```python
from build123d import *

# Parameters (mm, degrees)
SKETCH1_R            = 6.5
BOSS_EXTRUDE1_DEPTH  = 4
SKETCH4_R            = 2.6
CUT_EXTRUDE1_DEPTH   = 10
SKETCH5_W            = 200
SKETCH5_H            = 4
BOSS_EXTRUDE2_DEPTH  = 100
SKETCH8_R            = 2.6
CUT_EXTRUDE2_DEPTH   = 100
SKETCH9_R            = 5
SKETCH9_R_2          = 1.75
CUT_EXTRUDE3_DEPTH   = 10
CONVERT_SOLID3_START = -100
CONVERT_SOLID3_DEPTH = 200
SKETCH11_R           = 2.6
CUT_EXTRUDE4_DEPTH   = 10


# Read off the part's stored shape, not the designer's step: Convert-Solid3
with BuildPart() as part:
    # Sketch1 → Boss-Extrude1 (new body)
    with BuildSketch(Plane.XY):
        with BuildLine():
            Line((100, -4), (100, 0))
            Line((100, 0), (36.695562583, 145.919663525))
            ThreePointArc((36.695562583, 145.919663525), (0, 170), (-36.695562583, 145.919663525))
            Line((-36.695562583, 145.919663525), (-100, 0))
            Line((-100, 0), (-100, -4))
            Line((-100, -4), (100, -4))
        make_face()
        with Locations((0, 130)):
            Circle(SKETCH1_R, mode=Mode.SUBTRACT)
    extrude(amount=BOSS_EXTRUDE1_DEPTH)

    # Sketch4 → Cut-Extrude1 (cut)
    with BuildSketch(Plane(origin=(0, 0, 0), x_dir=(-1, 0, 0), z_dir=(0, 0, -1))):
        with Locations((0, 111.75)):
            Circle(SKETCH4_R)
        with Locations((0, 148.25)):
            Circle(SKETCH4_R)
    extrude(amount=-CUT_EXTRUDE1_DEPTH, mode=Mode.SUBTRACT)

    # Sketch5 → Boss-Extrude2 (add)
    with BuildSketch(Plane(origin=(0, 0, 0), x_dir=(-1, 0, 0), z_dir=(0, 0, -1))):
        with Locations((0, -2)):
            Rectangle(SKETCH5_W, SKETCH5_H)
    extrude(amount=-BOSS_EXTRUDE2_DEPTH)

    # Sketch8 → Cut-Extrude2 (cut)
    with BuildSketch(Plane(origin=(0, 0, 0), x_dir=(1, 0, 0), z_dir=(0, 1, 0))):
        with Locations(Location((-85, -80, 0), (0, 0, 270))):
            Circle(SKETCH8_R)
        with Locations(Location((-85, -20, 0), (0, 0, 270))):
            Circle(SKETCH8_R)
        with Locations(Location((85, -80, 0), (0, 0, 270))):
            Circle(SKETCH8_R)
        with Locations(Location((85, -20, 0), (0, 0, 270))):
            Circle(SKETCH8_R)
    extrude(amount=-CUT_EXTRUDE2_DEPTH, mode=Mode.SUBTRACT)

    # Sketch9 → Cut-Extrude3 (cut)
    with BuildSketch(Plane.XY.offset(4)):
        with Locations((0, 25)):
            Circle(SKETCH9_R)
        with Locations((0, 33)):
            Circle(SKETCH9_R_2)
        with Locations((0, 17)):
            Circle(SKETCH9_R_2)
        with Locations((8, 25)):
            Circle(SKETCH9_R_2)
        with Locations((-8, 25)):
            Circle(SKETCH9_R_2)
    extrude(amount=-CUT_EXTRUDE3_DEPTH, mode=Mode.SUBTRACT)

    # Convert-Solid3 outline → Convert-Solid3 (cut)
    with BuildSketch(Plane.YZ.offset(CONVERT_SOLID3_START)):
        with BuildLine():
            ThreePointArc((-0.2, 0), (-2.887005769, 1.112994231), (-4, 3.8))
            Line((-4, 3.8), (-3.999999957, 100))
            Line((-3.999999957, 100), (-6, 100))
            Line((-6, 100), (-6, -1))
            Line((-6, -1), (171, -1))
            Line((171, -1), (171, 7.6e-08))
            Line((171, 7.6e-08), (-0.2, 0))
        make_face()
        with BuildLine():
            Line((0, 100), (-2, 100))
            Line((-2, 100), (-2, 3.8))
            ThreePointArc((-2, 3.8), (-1.472792206, 2.527207794), (-0.2, 2))
            Line((-0.2, 2), (171, 2))
            Line((171, 2), (171, 4))
            Line((171, 4), (0, 4))
            Line((0, 4), (0, 100))
        make_face()
    extrude(amount=CONVERT_SOLID3_DEPTH, mode=Mode.SUBTRACT)

    # Sketch11 → Cut-Extrude4 (cut)
    with BuildSketch(Plane.XY.offset(2)):
        with Locations((0, 70)):
            Circle(SKETCH11_R)
        with Locations((0, 96.75)):
            Circle(SKETCH11_R)
        with Locations((-15, 96.75)):
            Circle(SKETCH11_R)
        with Locations((-15, 70)):
            Circle(SKETCH11_R)
    extrude(amount=-CUT_EXTRUDE4_DEPTH, mode=Mode.SUBTRACT)


solid = part.part
```
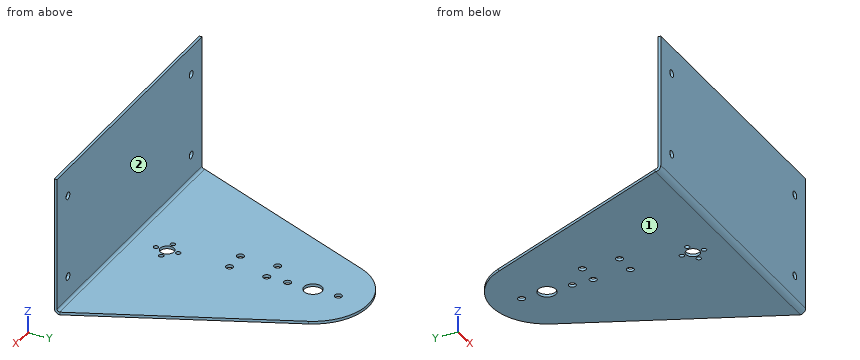
Geometry: final body of the model. Coordinates: model frame, mm. Face numbers are marked on the shaded views. A direction names the side the tool comes from. Coordinates: 2 decimals unless noted, no trailing zeros. Order: outer loops, then holes, each group sorted by start corner. A loop starts at its lowest first (then second) coordinate and runs counter-clockwise, first axis right, second up.
Item 1: Material intervals for line 1 along X through (y, z) = (-3.35, 20); line 2 along Y through (x, z) = (-15, 0.5); line 3 along Y through (x, z) = (-15, 1), sorted ascending.
Answer:
line 1: x = -100 to -87.6, -82.4 to 82.4, 87.6 to 100
line 2: y = -2.08 to 67.4, 72.6 to 94.15, 99.35 to 167.08
line 3: y = -2.77 to 67.4, 72.6 to 94.15, 99.35 to 167.08
Item 2: Contact query for flat-ended pins moving along their axis: P1, Ø6, axis at x = -15, y = 96.75, coming from the +Z side; P2, Ø10, axis at x = 22, z = 30.5, coming from the +Y side. Output: stop coordinate, or through.
Answer:
P1: stops at z = 2
P2: stops at y = -2
Item 3: Section query D-D (x = 85). Output: boundary loops of the cut face in (y, z), then the cut area to 3 significant figures.
Answer:
outline: (-4, 3.8) arc R3.8 ccw to (-0.2, 0) - (34.58, 0) - (34.58, 2) - (-0.2, 2) arc R1.8 cw to (-2, 3.8) - (-2, 17.4) - (-4, 17.4) - close; (-4, 22.6) - (-2, 22.6) - (-2, 77.4) - (-4, 77.4) - close; (-4, 82.6) - (-2, 82.6) - (-2, 100) - (-4, 100) - close
area: 250 mm2
Item 4: Section query A-A (y = 148.25). Output: boundary loops of the cut face in (x, z), then the cut area to 3 significant figures.
Answer:
outline: (-35.59, 0) - (-2.6, 0) - (-2.6, 2) - (-35.59, 2) - close; (2.6, 0) - (35.59, 0) - (35.59, 2) - (2.6, 2) - close
area: 132 mm2
Item 5: Section query B-B (x = -15). Output: boundary loops of the cut face in (y, z), then the cut area to 3 significant figures.
Answer:
outline: (-4, 3.8) arc R3.8 ccw to (-0.2, 0) - (67.4, 0) - (67.4, 2) - (-0.2, 2) arc R1.8 cw to (-2, 3.8) - (-2, 100) - (-4, 100) - close; (72.6, 0) - (94.15, 0) - (94.15, 2) - (72.6, 2) - close; (99.35, 0) - (167.08, 0) - (167.08, 2) - (99.35, 2) - close
area: 515 mm2
Item 6: Section query C-C (z = 30.5). Output: boundary loops of the cut face in (x, y), then the cut area to 3 significant figures.
Answer:
outline: (-100, -4) - (100, -4) - (100, -2) - (-100, -2) - close
area: 400 mm2
Item 7: Access query for the marked faces 1 and 2. Directions: +Z, -Z, +X, -X, +Y, -Y. A direction counts if a zero-diameter tool reaches every point of the face in a straight line with its end or side. Return the directions, or none.
Answer:
face 1: -Z, +X, -X, +Y, -Y
face 2: +Z, +X, -X, +Y
